Answer from the drawing. Dimensions are ordinates in mm from the lowest x, y and z of the part. A direction names the side the tool comes from. Give positions to 0.01 mm unless a question says otherwise; leave off trailing zeros. Write each loop counter-clockwise with the first axis right and the second up, starting at its lowest first coordinate (ties: lowest second). Pieces come first, ordered by that corner, then holes. Notation, with made-up numbers: (45, -27.5) -> (53, -27.5) arc R32 ccw to (53, -1.5) -> close; hole circle Ø9 at (-4.5, 46.5). An arc over 180 degrees is marked (long way). Use a Markdown table: item, result. Add a question column.
Q1. Section C-C, the plane x = 21 is taken. Give the vertices of the cut face in (y, z), plus the area to 3 significant figures.
Q2. Consider line 1 (X direction, y = 6.25, z = 4.5); line 2 (Y direction, x = 20.5, z = 30.5); line 3 (X direction, y = 14, z = 12). Determine where each line is inside the solid, lowest interval first.
Q3. Section B-B, the plane y = 4 is taken. Give the vertices of the cut face in (x, z), plus the area to 3 significant figures.
Q4. For a pull along Y with two mould halves and no side action, classify the marked faces 3, 4 and 5 as pulls with the +Y half, pulls with the -Y half, needs draft (parallel to the pull), parting line crosses it, or undercut.
Q5. Each of these flat-tipped pins is pushed along its axis until it touches: pin 1 Ø2 at (y, z) = (13.5, 21.5) entering from -X; pin 2 Ø5.5 at (y, z) = (9, 12) entering from +X. Where does it stop, or does it pass through?
Q6. Section A-A, the plane z = 12 is taken. Give the vertices of the cut face in (x, y).
Q7. For the marked faces 1 and 2, determine the directions among +Z, -Z, +X, -X, +Y, -Y from which every point of the face is accessible in a straight line to the end or side of a thin tool.
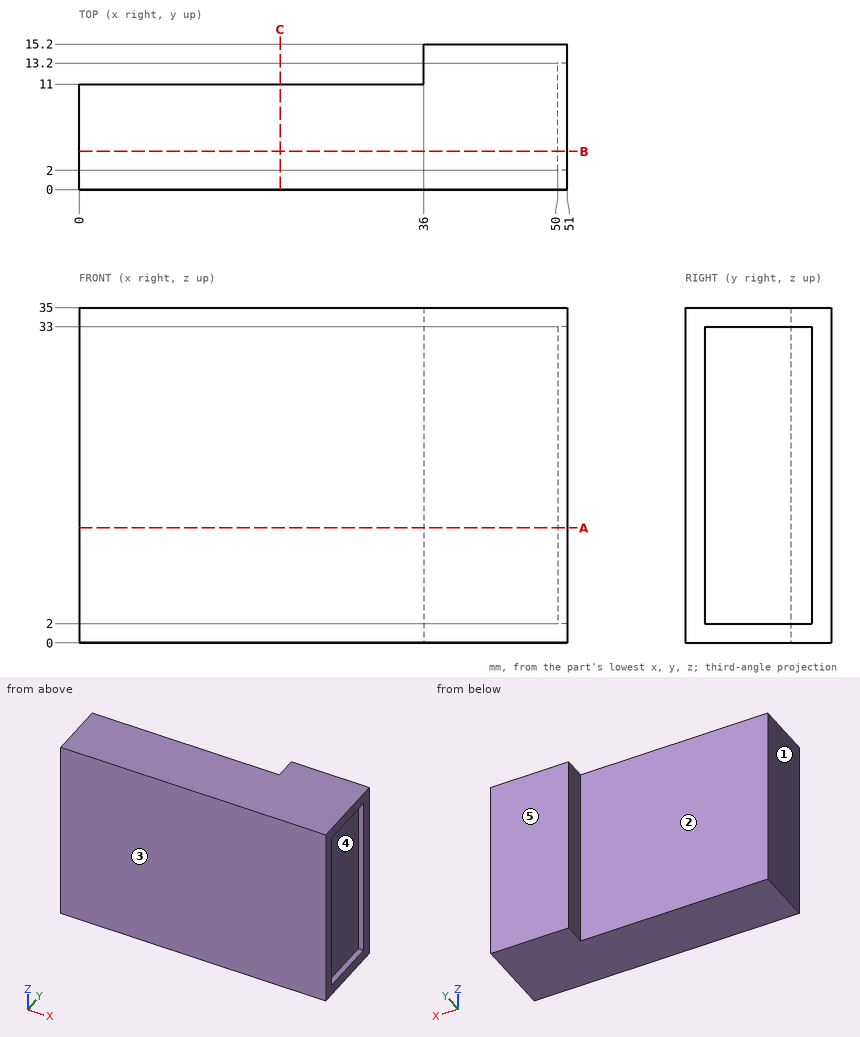
Result set:
| question | item | result |
|---|---|---|
| 1 | outline | (0, 0) -> (11, 0) -> (11, 35) -> (0, 35) -> close |
| 1 | area | 385 mm2 |
| 2 | line 1 | x = 0 to 50 |
| 2 | line 2 | y = 0 to 11 |
| 2 | line 3 | x = 36 to 51 |
| 3 | outline | (0, 0) -> (51, 0) -> (51, 2) -> (50, 2) -> (50, 33) -> (51, 33) -> (51, 35) -> (0, 35) -> close |
| 3 | area | 1,750 mm2 |
| 4 | face 3 | pulls with the -Y half |
| 4 | face 4 | undercut |
| 4 | face 5 | pulls with the +Y half |
| 5 | pin 1 | stops at x = 36 |
| 5 | pin 2 | stops at x = 50 |
| 6 | outline | (0, 0) -> (51, 0) -> (51, 2) -> (50, 2) -> (50, 13.2) -> (51, 13.2) -> (51, 15.2) -> (36, 15.2) -> (36, 11) -> (0, 11) -> close |
| 7 | face 1 | +Z, -Z, -X, +Y, -Y |
| 7 | face 2 | +Z, -Z, -X, +Y |
